Drawing for the job (mm, zero at the part's lowest x, y, z). Round coordinates to 2 decimals unless told otherwise and drop trailing zeros. Order: outer loops, then holes, each group sorted by start corner. A loop starts at its lowest first (then second) coordinate and runs counter-clockwise, first axis right, second up. Notation, with made-up numbers: (-30, 19) - (-2, 19) arc R29 ccw to (-2, 42) - close; hole circle Ø8 at (18.25, -11). An arc over 180 degrees is marked (long way). One line per question, with ' | ' between items. Start each with the question number.
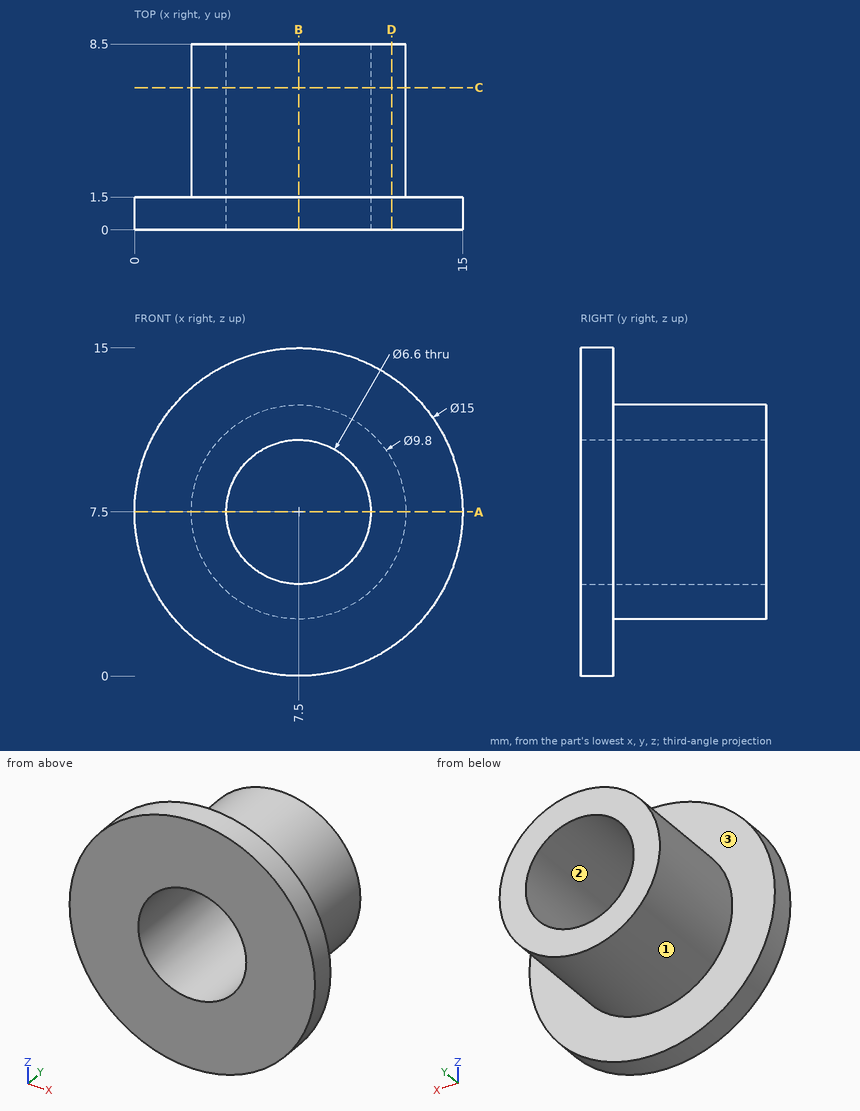
Item 1: Wall check: line 1 along Z through (x, y) = (7.5, 4.25); line 2 along Y through (x, z) = (8.75, 2.5). Give the ranges that are in metal, low to high. Write a range as [from, to].
Item 2: Slice it at B-B (x = 7.5). Write the cut outline in (y, z).
Item 3: Slice it at C-C (y = 6.5). Write the cut outline in (x, z), plus the area to 3 significant figures.
Item 4: Slice it at D-D (x = 11.75). Write the cut outline in (y, z).
Item 5: Pin check, flat tip, straight feed: pin 1 (5 mm diameter, centred on x = 5, z = 6, fed in from -Y). Stop position of the tip, or through.
Item 6: Pull direction X, two halves, no side cores. Call the marked faces 1, 2 and 3: released by +X, released by -X, zero draft, split by the parting line, or undercut.
Item 7: Slice it at A-A (z = 7.5). Write the cut outline in (x, y).
A:
1) line 1: [2.6, 4.2], [10.8, 12.4] | line 2: [0, 1.5]
2) outline: (0, 0) - (1.5, 0) - (1.5, 2.6) - (8.5, 2.6) - (8.5, 4.2) - (0, 4.2) - close; (0, 10.8) - (8.5, 10.8) - (8.5, 12.4) - (1.5, 12.4) - (1.5, 15) - (0, 15) - close
3) outline: circle Ø9.8 at (7.5, 7.5); hole circle Ø6.6 at (7.5, 7.5) | area: 41.2 mm^2
4) outline: (0, 1.32) - (1.5, 1.32) - (1.5, 5.06) - (8.5, 5.06) - (8.5, 9.94) - (1.5, 9.94) - (1.5, 13.68) - (0, 13.68) - close
5) pin 1: y = 0
6) face 1: split by the parting line | face 2: undercut | face 3: zero draft
7) outline: (0, 0) - (4.2, 0) - (4.2, 8.5) - (2.6, 8.5) - (2.6, 1.5) - (0, 1.5) - close; (10.8, 0) - (15, 0) - (15, 1.5) - (12.4, 1.5) - (12.4, 8.5) - (10.8, 8.5) - close
